```python
from build123d import *

# Parameters (mm, degrees)
SKETCH_1_W          = 5
SKETCH_1_H          = 25
SKETCH_1_R          = 1
EXTRUDE_1_DEPTH     = 2.5
SKETCH_3_W          = 5
SKETCH_3_H          = 15
EXTRUDE_2_DEPTH     = 20
SKETCH_6_W          = 9
SKETCH_6_H          = 20
CUT_EXTRUDE_1_DEPTH = 27.220221204
EXTRUDE_3_DEPTH     = 5


with BuildPart() as part:
    # 草图1 → 凸台-拉伸1 (new body)
    with BuildSketch(Plane(origin=(0, 0, 0), x_dir=(1, 0, 0), z_dir=(0, 1, 0))):
        Rectangle(SKETCH_1_W, SKETCH_1_H)
        with Locations(Location((0, 10, 0), (0, 0, 270))):
            Circle(SKETCH_1_R, mode=Mode.SUBTRACT)
        with Locations(Location((0, -10, 0), (0, 0, 90))):
            Circle(SKETCH_1_R, mode=Mode.SUBTRACT)
    extrude(amount=EXTRUDE_1_DEPTH)

    # 草图3 → 凸台-拉伸2 (add)
    with BuildSketch(Plane(origin=(0, 2.5, 0), x_dir=(1, 0, 0), z_dir=(0, 1, 0))):
        Rectangle(SKETCH_3_W, SKETCH_3_H)
    extrude(amount=EXTRUDE_2_DEPTH)

    # 草图6 → 切除-拉伸1 (cut, through all)
    with BuildSketch(Plane(origin=(2.5, 0, 0), x_dir=(0, 0, -1), z_dir=(1, 0, 0))):
        with Locations((0, 12.5)):
            Rectangle(SKETCH_6_W, SKETCH_6_H)
    extrude(amount=-CUT_EXTRUDE_1_DEPTH, mode=Mode.SUBTRACT)

    # 草图5 → 凸台-拉伸3 (add)
    with BuildSketch(Plane(origin=(2.5, 0, 0), x_dir=(0, 0, -1), z_dir=(1, 0, 0))):
        Polygon((-7.5, 15.011970436), (-10.454423259, 15.532914969), (-10.454423259, 18.532914969), (-7.5, 22.5), align=None)
    extrude(amount=-EXTRUDE_3_DEPTH)


solid = part.part
```
CAD build for the part. Positions are in the model's coordinates, mm. A direction names the side the tool comes from. Round coordinates to 2 decimals unless told otherwise and drop trailing zeros. Write each loop counter-clockwise with the first axis right and the second up, starting at its lowest first coordinate (ties: lowest second). Pieces come first, ordered by that corner, then holes. Notation, with made-up numbers: (41.5, 79) - (91.5, 79) arc R21 ccw to (91.5, 92) - close; hole circle Ø6 at (-30, -28.75). An arc over 180 degrees is marked (long way). Write item = value, one per line. Start each with the question number.
Q1. Band-saw the part on D-D (x = -1.45). Give the cut face in (y, z).
Q2. Mould opens along Z. For faces 1 (the flat face through (0, 1, -12.5)), 2 (the cylindrical face through (-0.6, 1.2, -10.8)), 3 (the flat face through (0, 12, -4.5)), 4 (the flat face through (-2.5, 10, 5)) say: pulls with the +Z half, pulls with the -Z half, needs draft (parallel to the pull), parting line crosses it, or undercut.
Q3. Band-saw the part on A-A (z = -10). Give the cut face in (x, y), then the cut area to 3 significant figures.
Q4. Probe L1, parallel to Z at x = -0.1, y = 12.5; L2, parallel to X at y = 1.95, z = 10; L3, parallel to Y at x = 1.9, z = 2.75. List the from-to ranges inside material, lowest first. Write a range as from..to.
Q5. Drop flat-ended pins along their axis: pin 1 (1 mm diameter, centred on x = -0.5, z = 1.5, fed in from -Y); pin 2 (1 mm diameter, centred on x = -2, y = 10.5, fed in from +Z); pin 3 (2.5 mm diameter, centred on x = -0.5, z = 10.5, fed in from +Y); pin 4 (1 mm diameter, centred on x = 1, z = -0.5, fed in from +Y). Give the stop position or say it passes through.
Q6. Band-saw the part on B-B (y = 8.5). Give the cut face in (x, z).
Q7. Which spindle directions (+Z, -Z, +X, -X, +Y, -Y) get a long thin tool onto all of the face, cutting with end or side? Do faces 5 (the flat face through (0, 17, 10.454)), 6 (the flat face through (0, 12, -7.5)), 7 (the flat face through (-0.03, 2.5, 8.85)), 8 (the flat face through (0, 2.5, 0)), 9 (the cylindrical face through (0.6, 1.2, 10.8)). Say none if no direction does.
Q8. Band-saw the part on C-C (x = 0). Give the cut face in (y, z), then the cut area to 3 significant figures.
Answers below:
q1.outline = (0, -12.5) - (2.5, -12.5) - (2.5, -7.5) - (22.5, -7.5) - (22.5, -4.5) - (2.5, -4.5) - (2.5, 4.5) - (22.5, 4.5) - (22.5, 7.5) - (18.53, 10.45) - (15.53, 10.45) - (15.01, 7.5) - (2.5, 7.5) - (2.5, 12.5) - (0, 12.5) - close
q2.face_1 = pulls with the -Z half
q2.face_2 = undercut
q2.face_3 = undercut
q2.face_4 = needs draft
q3.outline = (-2.5, 0) - (-1, 0) - (-1, 2.5) - (-2.5, 2.5) - close; (1, 0) - (2.5, 0) - (2.5, 2.5) - (1, 2.5) - close
q3.area = 7.50 mm2
q4.L1 = -7.5..-4.5, 4.5..7.5
q4.L2 = -2.5..-1, 1..2.5
q4.L3 = 0..2.5
q5.pin_1 = 0
q5.pin_2 = 7.5
q5.pin_3 = 20.15
q5.pin_4 = 2.5
q6.outline = (-2.5, -7.5) - (2.5, -7.5) - (2.5, -4.5) - (-2.5, -4.5) - close; (-2.5, 4.5) - (2.5, 4.5) - (2.5, 7.5) - (-2.5, 7.5) - close
q7.face_5 = +Z, +X, -X, +Y
q7.face_6 = -Z, +X, -X, +Y
q7.face_7 = +Z, +X, -X
q7.face_8 = +X, -X, +Y
q7.face_9 = -Y
q8.outline = (0, -12.5) - (2.5, -12.5) - (2.5, -11) - (0, -11) - close; (0, -9) - (2.5, -9) - (2.5, -7.5) - (22.5, -7.5) - (22.5, -4.5) - (2.5, -4.5) - (2.5, 4.5) - (22.5, 4.5) - (22.5, 7.5) - (18.53, 10.45) - (15.53, 10.45) - (15.01, 7.5) - (2.5, 7.5) - (2.5, 9) - (0, 9) - close; (0, 11) - (2.5, 11) - (2.5, 12.5) - (0, 12.5) - close
q8.area = 188 mm2
